Read the model definition and answer for the solid it produces. Units are mm, in the model's axes. A direction names the side the tool comes from. Coordinates: 2 decimals unless noted, no trailing zeros. Order: outer loops, then holes, each group sorted by start corner. A loop starts at its lowest first (then second) coordinate and runs counter-clockwise, first axis right, second up. Notation, with made-up numbers: (17.5, 55.5) -> (42.5, 55.5) arc R6 ccw to (42.5, 60.5) -> close; hole circle Ø2 at (31, -9). An arc over 180 degrees is marked (long way). Return JSON: item names as keys, results as strings. Group by question number.
```python
from build123d import *

# Parameters (mm, degrees)
SKETCH_1_R               = 27.5
EXTRUDE_1_DEPTH          = 5
SKETCH_2_R               = 10
CUT_EXTRUDE_2_DEPTH      = 6
SKETCH_2_12_R            = 16
SKETCH_2_12_R_2          = 10
EXTRUDE_9_DEPTH          = 15
SKETCH_12_R              = 2
CUT_EXTRUDE_3_DEPTH      = 6
CHAMFER_1_SIZE           = 0.5
CUT_EXTRUDE_START        = -6.202041
SKETCH_13_R              = 2
CUT_EXTRUDE_4_DEPTH      = 6.202041
PATTERN_CIRCULAR_1_COUNT = 4


with BuildPart() as part:
    # Sketch 1 → Extrude 1 (new body)
    with BuildSketch(Plane.XY):
        Circle(SKETCH_1_R)
    extrude(amount=EXTRUDE_1_DEPTH)

    # Sketch 2 → Cut-Extrude 2 (cut, through all)
    with BuildSketch(Plane(origin=(0, 0, 0), x_dir=(-1, 0, 0), z_dir=(0, 0, -1))):
        Circle(SKETCH_2_R)
    extrude(amount=-CUT_EXTRUDE_2_DEPTH, mode=Mode.SUBTRACT)

    # Sketch 2_12 → Extrude 9 (add)
    with BuildSketch(Plane(origin=(0, 0, 0), x_dir=(-1, 0, 0), z_dir=(0, 0, -1))):
        Circle(SKETCH_2_12_R)
        Circle(SKETCH_2_12_R_2, mode=Mode.SUBTRACT)
    extrude(amount=EXTRUDE_9_DEPTH)

    # Sketch 12 → Cut-Extrude 3 (cut, through all)
    with BuildSketch(Plane(origin=(0, 0, 0), x_dir=(-1, 0, 0), z_dir=(0, 0, -1))):
        with Locations((-22.5, 0)):
            Circle(SKETCH_12_R)
        with Locations((-11.25, 19.485571585)):
            Circle(SKETCH_12_R)
        with Locations((11.25, 19.485571585)):
            Circle(SKETCH_12_R)
        with Locations((22.5, 0)):
            Circle(SKETCH_12_R)
        with Locations((11.25, -19.485571585)):
            Circle(SKETCH_12_R)
        with Locations((-11.25, -19.485571585)):
            Circle(SKETCH_12_R)
    extrude(amount=-CUT_EXTRUDE_3_DEPTH, mode=Mode.SUBTRACT)

    # Chamfer 1
    chamfer_1_edges = [part.edges().sort_by_distance(p)[0] for p in [
        (-20.5, 0, 0),
        (-9.25, -19.485571585, 0),
        (13.25, -19.485571585, 0),
        (24.5, 0, 0),
        (13.25, 19.485571585, 0),
        (-9.25, 19.485571585, 0),
    ]]
    chamfer(chamfer_1_edges, length=CHAMFER_1_SIZE)

    # Sketch 13 → Cut-Extrude 4 (cut)
    with BuildSketch(Plane(origin=(0, 16, 0), x_dir=(1, 0, 0), z_dir=(0, 1, 0)).offset(CUT_EXTRUDE_START)):
        with Locations((0, 7.5)):
            Circle(SKETCH_13_R)
    cut_extrude_4 = extrude(amount=CUT_EXTRUDE_4_DEPTH, mode=Mode.SUBTRACT)

    # Pattern Circular 1: Cut-Extrude 4 ×4 about axis
    pattern_circular_1_axis = Axis((0, 0, -15), (0, 0, 1))
    for i in range(1, PATTERN_CIRCULAR_1_COUNT):
        add(cut_extrude_4.rotate(pattern_circular_1_axis, i * 360 / PATTERN_CIRCULAR_1_COUNT), mode=Mode.SUBTRACT)


solid = part.part
```
1. Find section A-A on x = 0. Determine the outline of the cut face in (y, z), and give its area (3 significant figures).
2. Find section D-D on z = -7.5. Determine the outline of the cut face in (x, y).
3. Find section B-B on y = 0. Give the number of separate pieces and of enclosed holes in the cut face, and give its area (4 significant figures).
4. Find section C-C on x = 11.25. Determine the outline of the cut face in (y, z), and give its area (3 significant figures).
5. Which of the six approach directions +Z, -Z, +X, -X, +Y, -Y give full straight-line access (tool end or side, diameter ignored) to faces 1 (the face through (0.26, -12.855, -9.483)), 2 (the face through (12, -12, 0))?
6. Given pin 1 (2 mm diameter, centred on y = -14.5, z = 1.5, fed in from +X); pin 2 (5 mm diameter, centred on y = 0, z = -7.5, fed in from -X); pin 3 (4 mm diameter, centred on x = -5, z = -4, fed in from +Y), each flat-ended and moving along its own axis, determine where each tip first touches the part or whether it passes through.
7. Straight lines are drawn through the part: L1, parallel to Y at x = -11.25, z = 1.9; L2, parallel to Z at x = 18, y = 7; L3, parallel to Z at x = 0, y = 12. For each, find the intervals that lie inside material, in ascending order.
8. For a pull along Z with two mould halves and no side action, classify faces 3 (the face through (-0.26, 12.855, -9.483)), 4 (the face through (-9.25, 19.57, 2.72)), 5 (the face through (-10.4, 0.2, -15)) as released by +Z, released by -Z, zero draft, split by the parting line, or undercut.
Result:
{
 "1": {"outline": "(-27.5, 0) -> (-16, 0) -> (-16, -5.5) -> (-10, -5.5) -> (-10, 5) -> (-27.5, 5) -> close; (-16, -15) -> (-10, -15) -> (-10, -9.5) -> (-16, -9.5) -> close; (10, -15) -> (16, -15) -> (16, -9.5) -> (10, -9.5) -> close; (10, -5.5) -> (16, -5.5) -> (16, 0) -> (27.5, 0) -> (27.5, 5) -> (10, 5) -> close", "area": "307 mm^2"},
 "2": {"outline": "(-15.87, -2) arc R16 ccw to (-2, -15.87) -> (-2, -9.8) arc R10 cw to (-9.8, -2) -> close; (-15.87, 2) -> (-9.8, 2) arc R10 cw to (-2, 9.8) -> (-2, 15.87) arc R16 ccw to start; (2, -15.87) arc R16 ccw to (15.87, -2) -> (9.8, -2) arc R10 cw to (2, -9.8) -> close; (2, 9.8) arc R10 cw to (9.8, 2) -> (15.87, 2) arc R16 ccw to (2, 15.87) -> close"},
 "3": {"separate pieces": "6", "enclosed holes": "0", "area": "266.5 mm^2"},
 "4": {"outline": "(-25.09, 0) -> (-21.99, 0) -> (-21.49, 0.5) -> (-21.49, 5) -> (-25.09, 5) -> close; (-17.49, 0.5) -> (-16.99, 0) -> (-11.38, 0) -> (-11.38, -15) -> (11.38, -15) -> (11.38, 0) -> (16.99, 0) -> (17.49, 0.5) -> (17.49, 5) -> (-17.49, 5) -> close; (21.49, 0.5) -> (21.99, 0) -> (25.09, 0) -> (25.09, 5) -> (21.49, 5) -> close; hole circle Ø4 at (0, -7.5)", "area": "539 mm^2"},
 "5": {"face 1": "+Y, -Y", "face 2": "-Z"},
 "6": {"pin 1": "x = 23.96", "pin 2": "x = -16", "pin 3": "y = 15.72"},
 "7": {"L1": "-25.09 to -21.49, -17.49 to 17.49, 21.49 to 25.09", "L2": "0 to 5", "L3": "-15 to -9.5, -5.5 to 5"},
 "8": {"face 3": "undercut", "face 4": "zero draft", "face 5": "released by -Z"}
}
